Build history of the part. All positions in model axes, mm. Round coordinates to 2 decimals unless told otherwise and drop trailing zeros. Write each loop counter-clockwise with the first axis right and the second up, starting at its lowest first coordinate (ties: lowest second). Pieces come first, ordered by that corner, then holes. Notation, with made-up numbers: M 66.25,60 L 117.25,60 A14 ccw 117.25,82 Z; hole C -3,-16.5 d2. An arc over 180 degrees is marked long. One line per item, written item: value. Start each with the question number.
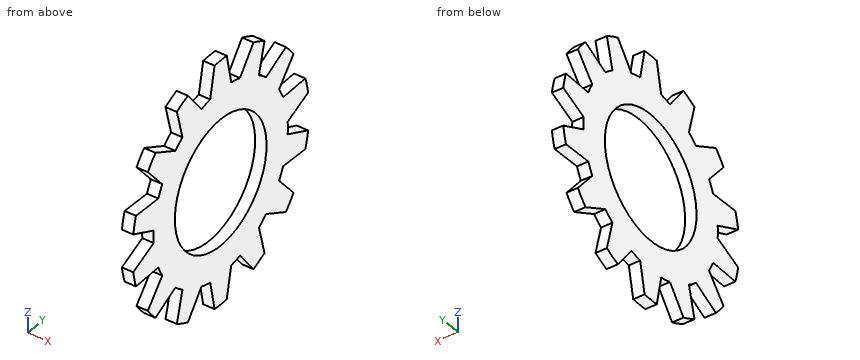
```python
from build123d import *

# Parameters (mm, degrees)
SECSKE_W      = 0.5842
SECSKE_H      = 3.0226
EXTCUT_DEPTH  = 9.891705265
EXTCUTS_COUNT = 14
EXTCUTS_ANGLE = 334.285714286


with BuildPart() as part:
    # SecSke → Body (revolve)
    with BuildSketch(Plane.XY, mode=Mode.PRIVATE) as body_sk:
        with Locations((-0.2921, 4.7625)):
            Rectangle(SECSKE_W, SECSKE_H)
    revolve(body_sk.sketch.rotate(Axis((-34.925, 0, 0), (1, 0, 0)), 90), axis=Axis((-34.925, 0, 0), (1, 0, 0)))

    # ExtCutSke → ExtCut (cut, through all)
    with BuildSketch(Plane(origin=(0, 0, 0), x_dir=(0, 0, -1), z_dir=(1, 0, 0))):
        with BuildLine():
            Line((-1.103445571, 6.494415476), (-0.320368639, 4.751712342))
            ThreePointArc((-0.320368639, 4.751712342), (0, 4.7625), (0.320368639, 4.751712342))
            Line((0.320368639, 4.751712342), (1.103445571, 6.494415476))
            ThreePointArc((1.103445571, 6.494415476), (0, 6.58749), (-1.103445571, 6.494415476))
        make_face()
    extcut = extrude(amount=-EXTCUT_DEPTH, mode=Mode.SUBTRACT)

    # ExtCuts: ExtCut ×14 about axis
    extcuts_axis = Axis((-34.925, 0, 0), (1, 0, 0))
    for i in range(1, EXTCUTS_COUNT):
        add(extcut.rotate(extcuts_axis, i * EXTCUTS_ANGLE / (EXTCUTS_COUNT - 1)), mode=Mode.SUBTRACT)


solid = part.part
```
Item 1: Cut at A-A, the plane z = 0. Write the cut outline in (x, y).
Item 2: Cut at C-C, the plane y = -5. Write the cut outline in (x, z), plus the area to 3 significant figures.
Item 3: Drill centre lines: line 1 (Y direction, x = -0.15, z = 3.75); line 2 (Y direction, x = -0.4, z = 0); line 3 (Y direction, x = -0.2, z = 1). Where is each one in solid material? Low to high.
Item 4: Cut at D-D, the plane y = 3.5. Write the cut outline in (x, z), plus the area to 3 significant figures.
Item 5: Cut at B-B, the plane y = 0. Write the cut outline in (x, z), plus the area to 3 significant figures.
Computed values:
1. outline: M -0.58,-4.76 L 0,-4.76 L 0,-3.25 L -0.58,-3.25 Z; M -0.58,3.25 L 0,3.25 L 0,4.76 L -0.58,4.76 Z
2. outline: M -0.58,-3.79 L 0,-3.79 L 0,-3.37 L -0.58,-3.37 Z; M -0.58,-1.79 L 0,-1.79 L 0,-0.43 L -0.58,-0.43 Z; M -0.58,0.43 L 0,0.43 L 0,1.79 L -0.58,1.79 Z; M -0.58,3.37 L 0,3.37 L 0,3.79 L -0.58,3.79 Z
2. area: 2.08 mm2
3. line 1: y = -5.03 to -3.67, -2.94 to 2.94, 3.67 to 5.03
3. line 2: y = -4.76 to -3.25, 3.25 to 4.76
3. line 3: y = -6.19 to -3.09, 3.09 to 6.19
4. outline: M -0.58,-3.66 L 0,-3.66 L 0,3.66 L -0.58,3.66 Z
4. area: 4.28 mm2
5. outline: M -0.58,-6.27 L 0,-6.27 L 0,-3.25 L -0.58,-3.25 Z; M -0.58,3.25 L 0,3.25 L 0,6.27 L -0.58,6.27 Z
5. area: 3.53 mm2
